from build123d import *

# Parameters (mm, degrees)
BOSS_EXTRUDE1_DEPTH          = 7
HOLE1_D                      = 8
HOLE1_CBORE_D                = 20.5
HOLE1_CBORE_DEPTH            = 2.5
F_1_0_1_DIAMETER_HOLE1_D     = 1
F_1_0_1_DIAMETER_HOLE1_DEPTH = 7


with BuildPart() as part:
    # Sketch1 → Boss-Extrude1 (new body)
    with BuildSketch(Plane(origin=(0, 0, 74.1), x_dir=(-1, 0, 0), z_dir=(0, 0, -1))):
        with BuildLine():
            Line((5.573417888, 7.249599077), (3.909244984, 5.703911435))
            ThreePointArc((3.909244984, 5.703911435), (3.809726926, 5.099679562), (4.369892407, 4.852263649))
            Line((4.369892407, 4.852263649), (6.574346511, 5.399076092))
            ThreePointArc((6.574346511, 5.399076092), (6.86485582, 4.975241994), (7.172578897, 4.563735604))
            Line((7.172578897, 4.563735604), (5.94508593, 2.65274561))
            ThreePointArc((5.94508593, 2.65274561), (5.998960771, 2.042747658), (6.603057459, 1.942412262))
            Line((6.603057459, 1.942412262), (8.602267858, 3.020271029))
            ThreePointArc((8.602267858, 3.020271029), (8.989053537, 2.681999186), (9.389446406, 2.359948643))
            Line((9.389446406, 2.359948643), (8.675761274, 0.203730826))
            ThreePointArc((8.675761274, 0.203730826), (8.87964386, -0.37370479), (9.489714138, -0.320655229))
            Line((9.489714138, -0.320655229), (11.158063091, 1.220524032))
            ThreePointArc((11.158063091, 1.220524032), (11.616821973, 0.989069307), (12.084726477, 0.776710232))
            Line((12.084726477, 0.776710232), (11.92969264, -1.489252312))
            ThreePointArc((11.92969264, -1.489252312), (12.270772279, -1.997843189), (12.848483188, -1.794741969))
            Line((12.848483188, -1.794741969), (14.081142194, 0.112919824))
            ThreePointArc((14.081142194, 0.112919824), (14.583048772, 0.00282537), (15.089064749, -0.086498936))
            Line((15.089064749, -0.086498936), (15.502423555, -2.319827447))
            ThreePointArc((15.502423555, -2.319827447), (15.959268957, -2.72761695), (16.468320796, -2.387225667))
            Line((16.468320796, -2.387225667), (17.187837357, -0.232946748))
            ThreePointArc((17.187837357, -0.232946748), (17.701354994, -0.214763292), (18.213687601, -0.175440255))
            Line((18.213687601, -0.175440255), (19.169466196, -2.235806489))
            ThreePointArc((19.169466196, -2.235806489), (19.713372085, -2.517171704), (20.121779254, -2.060878394))
            Line((20.121779254, -2.060878394), (20.282943498, 0.204656383))
            ThreePointArc((20.282943498, 0.204656383), (20.775805993, 0.349975216), (21.262263487, 0.515474786))
            Line((21.262263487, 0.515474786), (22.700406786, -1.242468784))
            ThreePointArc((22.700406786, -1.242468784), (23.297197554, -1.379730498), (23.57929833, -0.83620575))
            Line((23.57929833, -0.83620575), (23.171983715, 1.398233005))
            ThreePointArc((23.171983715, 1.398233005), (23.613222703, 1.661556297), (24.043239171, 1.942833453))
            Line((24.043239171, 1.942833453), (25.873383342, 0.597770608))
            ThreePointArc((25.873383342, 0.597770608), (26.485560432, 0.613237052), (26.623629384, 1.209841581))
            Line((26.623629384, 1.209841581), (25.673428985, 3.272786307))
            ThreePointArc((25.673428985, 3.272786307), (26.0353198, 3.637568488), (26.381875725, 4.016949552))
            Line((26.381875725, 4.016949552), (28.489026078, 3.169282677))
            ThreePointArc((28.489026078, 3.169282677), (29.078124151, 3.336505465), (29.063485901, 3.948702919))
            Line((29.063485901, 3.948702919), (27.630104303, 5.710531213))
            ThreePointArc((27.630104303, 5.710531213), (27.889908013, 6.153851676), (28.131228013, 6.607498741))
            Line((28.131228013, 6.607498741), (30.382984542, 6.310489863))
            ThreePointArc((30.382984542, 6.310489863), (30.911988399, 6.618961773), (30.745562721, 7.208285533))
            Line((30.745562721, 7.208285533), (28.919064562, 8.558295243))
            ThreePointArc((28.919064562, 8.558295243), (29.060456745, 9.052298535), (29.181377796, 9.551707286))
            Line((29.181377796, 9.551707286), (31.436254358, 9.824018565))
            ThreePointArc((31.436254358, 9.824018565), (31.871924741, 10.254357173), (31.564168772, 10.783777859))
            Line((31.564168772, 10.783777859), (29.459319649, 11.637142911))
            ThreePointArc((29.459319649, 11.637142911), (29.473416113, 12.150788987), (29.466340301, 12.664579737))
            Line((29.466340301, 12.664579737), (31.582654708, 13.489100854))
            ThreePointArc((31.582654708, 13.489100854), (31.897616846, 14.014266401), (31.467868026, 14.450518566))
            Line((31.467868026, 14.450518566), (29.21692335, 14.753618895))
            ThreePointArc((29.21692335, 14.753618895), (29.102838363, 15.254633483), (28.968210287, 15.750522868))
            Line((28.968210287, 15.750522868), (30.812986722, 17.07544613))
            ThreePointArc((30.812986722, 17.07544613), (30.987450384, 17.662440534), (30.462711412, 17.97811285))
            Line((30.462711412, 17.97811285), (28.207106316, 17.711903547))
            ThreePointArc((28.207106316, 17.711903547), (27.972008257, 18.168806058), (27.718287094, 18.615635525))
            Line((27.718287094, 18.615635525), (29.175611469, 20.357711129))
            ThreePointArc((29.175611469, 20.357711129), (29.198614462, 20.969651374), (28.611856617, 21.144908987))
            Line((28.611856617, 21.144908987), (26.493319064, 20.326116962))
            ThreePointArc((26.493319064, 20.326116962), (26.151980009, 20.710198531), (25.795107994, 21.079892141))
            Line((25.795107994, 21.079892141), (26.773411257, 23.129659071))
            ThreePointArc((26.773411257, 23.129659071), (26.643508219, 23.728094699), (26.031599654, 23.75192553))
            Line((26.031599654, 23.75192553), (24.183245151, 22.431998497))
            ThreePointArc((24.183245151, 22.431998497), (23.757112689, 22.719125866), (23.319513401, 22.988454411))
            Line((23.319513401, 22.988454411), (23.757325162, 25.217118272))
            ThreePointArc((23.757325162, 25.217118272), (23.482678378, 25.764447372), (22.88406756, 25.635354042))
            Line((22.88406756, 25.635354042), (21.422035016, 23.897227871))
            ThreePointArc((21.422035016, 23.897227871), (20.937884616, 24.069359772), (20.44705403, 24.221400348))
            Line((20.44705403, 24.221400348), (20.316864965, 26.488925992))
            ThreePointArc((20.316864965, 26.488925992), (19.914731502, 26.950757865), (19.367031349, 26.676851782))
            Line((19.367031349, 26.676851782), (18.383185648, 24.629739333))
            ThreePointArc((18.383185648, 24.629739333), (17.87143826, 24.676060085), (17.358217065, 24.701259423))
            Line((17.358217065, 24.701259423), (16.668207433, 26.865169876))
            ThreePointArc((16.668207433, 26.865169876), (16.163854816, 27.212485926), (15.701479344, 26.810977617))
            Line((15.701479344, 26.810977617), (15.257639128, 24.583506493))
            ThreePointArc((15.257639128, 24.583506493), (14.750449723, 24.501105593), (14.247085495, 24.397880327))
            Line((14.247085495, 24.397880327), (13.040611138, 26.322209137))
            ThreePointArc((13.040611138, 26.322209137), (12.465729697, 26.533186219), (12.117731656, 26.029303927))
            Line((12.117731656, 26.029303927), (12.241785039, 23.761434332))
            ThreePointArc((12.241785039, 23.761434332), (11.771022192, 23.555489332), (11.309143157, 23.330325485))
            Line((11.309143157, 23.330325485), (9.662011296, 24.894159994))
            ThreePointArc((9.662011296, 24.894159994), (9.052722946, 24.955541642), (8.840968333, 24.380946146))
            Line((8.840968333, 24.380946146), (9.525120585, 22.215176667))
            ThreePointArc((9.525120585, 22.215176667), (9.120364058, 21.898627848), (8.728991773, 21.565673292))
            Line((8.728991773, 21.565673292), (6.744697761, 22.670752028))
            ThreePointArc((6.744697761, 22.670752028), (6.139286329, 22.578681408), (6.077080467, 21.969476655))
            Line((6.077080467, 21.969476655), (7.278343785, 20.041890553))
            ThreePointArc((7.278343785, 20.041890553), (6.965025918, 19.634627842), (6.668751745, 19.214803336))
            Line((6.668751745, 19.214803336), (4.471976071, 19.791690138))
            ThreePointArc((4.471976071, 19.791690138), (3.908481786, 19.551952385), (3.999733295, 18.94641695))
            Line((3.999733295, 18.94641695), (5.642627888, 17.378131549))
            ThreePointArc((5.642627888, 17.378131549), (5.440435595, 16.905744761), (5.257875529, 16.425429423))
            Line((5.257875529, 16.425429423), (2.986649689, 16.43787637))
            ThreePointArc((2.986649689, 16.43787637), (2.500478968, 16.065535089), (2.739454182, 15.501716992))
            Line((2.739454182, 15.501716992), (4.72075094, 14.391273431))
            ThreePointArc((4.72075094, 14.391273431), (4.642388707, 13.883444364), (4.585013668, 13.372818174))
            Line((4.585013668, 13.372818174), (2.382047135, 12.820043179))
            ThreePointArc((2.382047135, 12.820043179), (2.003747871, 12.338493942), (2.375431099, 11.851819947))
            Line((2.375431099, 11.851819947), (4.570637859, 11.26899148))
            ThreePointArc((4.570637859, 11.26899148), (4.621029474, 10.757628901), (4.692444547, 10.24877638))
            Line((4.692444547, 10.24877638), (2.696157809, 9.16551233))
            ThreePointArc((2.696157809, 9.16551233), (2.449499938, 8.605012646), (2.930536955, 8.226062269))
            Line((2.930536955, 8.226062269), (5.201720804, 8.207470152))
            ThreePointArc((5.201720804, 8.207470152), (5.377699975, 7.724704854), (5.573417888, 7.249599077))
        make_face()
    extrude(amount=-BOSS_EXTRUDE1_DEPTH)

    # Hole1 (through all)
    with Locations(Plane(origin=(0, 0, 74.1), x_dir=(-1, 0, 0), z_dir=(0, 0, -1))):
        with Locations((17.003397692, 12.235998762)):
            CounterBoreHole(HOLE1_D / 2, HOLE1_CBORE_D / 2, HOLE1_CBORE_DEPTH)

    # Ø1.0 (1) Diameter Hole1
    with Locations(Plane.XY.offset(81.1)):
        with Locations((-13.846779088, 5.093992112), (-17.096499658, 5.136609209), (-20.346220228, 5.179226306), (-24.145404342, 9.079380158), (-24.102787245, 12.329100728), (-24.060170148, 15.578821298), (-20.160016296, 19.378005412), (-16.910295726, 19.335388315), (-13.660575156, 19.292771218), (-9.861391042, 15.392617366), (-9.904008139, 12.142896796), (-9.946625236, 8.893176226)):
            Hole(F_1_0_1_DIAMETER_HOLE1_D / 2, depth=F_1_0_1_DIAMETER_HOLE1_DEPTH)


solid = part.part
For this review, take the finished solid that the model builds, in its own axes (mm). A direction names the side the tool comes from. Give positions to 0.01 mm unless a question says otherwise; leave off trailing zeros. Answer as a JSON object with one key per item and string values. Group by question number.
Item 1: Machinability: for faces 5 (the flat face through (-29.351, 17.847, 77.551)), 6 (the flat face through (-28.357, 4.817, 77.551)), 7 (the flat face through (-18.685, -1.191, 77.551)), which of the approach directions +Z, -Z, +X, -X, +Y, -Y give a long, thin tool a straight path to every point of the face, cutting with its end or side? Answer none if there is none.
Item 2: Take a section at A-A on z = 80.5. Give the number of separate pieces and of enclosed holes in the cut face, and give its area (3 significant figures).
Item 3: Wall thickness on line 1 along X through (y, z) = (12, 79); line 2 along Y through (x, z) = (-28, 80.5); line 3 along Z through (x, y) = (-15.5, 18.75): over which ranges is each line inside the solid? List them lowest first.
Item 4: Draft analysis for pull direction Y (two halves, no side actions). For faces 1 (the flat face through (-13, 9, 81.1)), 2 (the cylindrical face through (-17.694, -0.215, 77.551)), 3 (the cylindrical face through (-31.87, 10.25, 77.55)), 4 (the flat face through (-18.882, 25.668, 77.551)), state which applies: pulls with the +Y half, pulls with the -Y half, needs draft (parallel to the pull), parting line crosses it, or undercut.
Item 5: Clearance check with flat-ended pins moving along their axes: pin 1 Ø4 at (x, z) = (-23, 75.5) entering from +Y; pin 2 Ø4 at (x, z) = (-7.5, 75.5) entering from -Y; pin 3 Ø4 at (y, z) = (18, 76.5) entering from -X. State where each tip first meets the part, or that it passes through.
Reported:
{
 "1": {"face 5": "+Z, -Z", "face 6": "+Z, -Z, -X", "face 7": "+Z, -Z, -Y"},
 "2": {"separate pieces": "1", "enclosed holes": "13", "area": "518 mm^2"},
 "3": {"line 1": "-29.47 to -24.48, -23.73 to -21, -13.01 to -10.38, -9.42 to -2.13", "line 2": "3.37 to 5.26, 6.36 to 18.12, 18.95 to 20.91", "line 3": "76.6 to 81.1"},
 "4": {"face 1": "needs draft", "face 2": "pulls with the -Y half", "face 3": "undercut", "face 4": "pulls with the +Y half"},
 "5": {"pin 1": "y = 25.81", "pin 2": "y = -0.45", "pin 3": "x = -31.02"}
}
